Source: CAD feature listing. Evaluate the final solid. Frame: model axes, mm. A direction names the side the tool comes from. Round coordinates to 2 decimals unless told otherwise and drop trailing zeros. Order: outer loops, then holes, each group sorted by start corner. A loop starts at its lowest first (then second) coordinate and runs counter-clockwise, first axis right, second up. Notation, with made-up numbers: (75, -27) - (124, -27) arc R20 ccw to (124, -22) - close; hole circle Ø10 at (-37.75, 27). An arc over 180 degrees is marked (long way). Put each result on its own line as item: value. Start each with the question number.
1) Section C-C on y = 4. Output: boundary loops of the cut face in (x, z).
2) Section D-D on x = -10.5. Output: boundary loops of the cut face in (y, z).
3) Mould query, pull axis Z, two halves, no side actions, for faces 1 (the face through (0, 7.62, -2)), 2 (the face through (-21, 4, 0)), 3 (the face through (-1.38, 3.76, -1.12)), 4 (the face through (0, 4, -6.35)). Classes: +Z half, -Z half, draft (parallel to the pull), parting line (faces both ways), or undercut.
4) Section A-A on z = 5.08. Output: boundary loops of the cut face in (x, y).
5) Line query: probe 1 along Z at (x, y) = (20, 7); probe 2 along X at (y, z) = (2.25, 5.08); probe 3 along X at (y, z) = (3.25, 9.25). Output: solid intervals per line, ascending. Write a range as [from, to].
6) Contact query for flat-ended pins moving along their axis: P1, Ø4, axis at x = -8.5, z = -2, coming from the -Y side; P2, Ø1.5, axis at y = 5, z = 10.5, coming from the +X side; P3, Ø3.5, axis at x = 20.5, y = 4.5, coming from the +Z side; P4, Ø1.5, axis at x = 10.5, y = 3, coming from the +Z side. Output: stop coordinate, or through.
7) Section B-B on x = -4.5. Output: boundary loops of the cut face in (y, z).
8) Access query for faces 5 (the face through (21, 4, 0)), 6 (the face through (-22.24, 4, -3)). Directions: +Z, -Z, +X, -X, +Y, -Y. A direction counts if a zero-diameter tool reaches every point of the face in a straight line with its end or side. Return the directions, or none.
Autodesk Fusion 360 part; units mm, degrees
sketch "Sketch1" plane through (0, 0, 0) normal (0, 1, 0) x (1, 0, 0)
  line L0 (-22.2401, 0) -> (22.2401, 0)
  line L1 (22.2401, 0) -> (22.2401, 6.35)
  line L2 (22.2401, 6.35) -> (-22.2401, 6.35)
  line L3 (-22.2401, 6.35) -> (-22.2401, 0)
  line L4 (0, 0) -> (0, -19.05)
  line L5 (0, -19.05) -> (-19.05, 0)
  line L6 (0, -19.05) -> (-21.997, -19.05) construction
  line L7 (0, -19.05) -> (19.05, 0)
  dimension "d1" = 19.05
  dimension "d2" = 45
  dimension "d6" = 25.4
extrude "Extrude1" add sketch "Sketch1" along normal blind 7.62
sketch "Sketch2" plane through (0, 0, 0) normal (0, -1, 0) x (1, 0, 0)
  line L0 (19.05, 0) -> (0, 19.05)
  line L1 (0, 19.05) -> (-19.05, 0)
  line L2 (-19.05, 0) -> (-22.2401, 0)
  line L3 (-22.2401, 0) -> (-22.2401, -6.35)
  line L4 (-22.2401, -6.35) -> (22.2401, -6.35)
  line L5 (22.2401, -6.35) -> (22.2401, 0)
  line L6 (22.2401, 0) -> (19.05, 0)
  line L7 (0, -6.35) -> (0, 20.8829)
  circle A0 centre (0, 5.08) radius 6.35
  dimension "d12" = 12.7
extrude "Extrude2" cut sketch "Sketch2" against normal blind 54.61 contours L7 A0 | L7 A0
equation "d1 = triangleHeight"
equation "d2 = triangleDeg"
equation "length = 1 in"
equation "height = 1 in"
equation "triangleHeight = 0.75 in"
equation "d6 = height"
equation "triangleDeg = 45 deg"
equation "width = 0.3 in"
equation "d9 = width"
equation "AxleHoleDia = 0.5 in"
equation "d12 = AxleHoleDia"
Answer sheet:
1. outline: (-22.24, -6.35) - (22.24, -6.35) - (22.24, 0) - (19.05, 0) - (0, 19.05) - (-19.05, 0) - (-22.24, 0) - close; hole circle Ø12.7 at (0, 5.08)
2. outline: (0, -6.35) - (7.62, -6.35) - (7.62, 8.55) - (0, 8.55) - close
3. face 1: draft
3. face 2: +Z half
3. face 3: undercut
3. face 4: -Z half
4. outline: (-13.97, 0) - (-6.35, 0) - (-6.35, 7.62) - (-13.97, 7.62) - close; (6.35, 0) - (13.97, 0) - (13.97, 7.62) - (6.35, 7.62) - close
5. probe 1: [-6.35, 0]
5. probe 2: [-13.97, -6.35], [6.35, 13.97]
5. probe 3: [-9.8, -4.79], [4.79, 9.8]
6. P1: y = 0
6. P2: x = 9.3
6. P3: z = 0.3
6. P4: z = 9.3
7. outline: (0, -6.35) - (7.62, -6.35) - (7.62, 0.6) - (0, 0.6) - close; (0, 9.56) - (7.62, 9.56) - (7.62, 14.55) - (0, 14.55) - close
8. face 5: +Z, +X, +Y, -Y
8. face 6: +Z, -Z, -X, +Y, -Y
